Geometry check sheet. Reference: drawing and pictorial views, mm from the part's lowest x, y, z. A direction names the side the tool comes from. Coordinates: 2 decimals unless noted, no trailing zeros. Loops run counter-clockwise (first coordinate to the right, second up) from the corner with the lowest first, then second, coordinate; pieces in that order, holes last. Notation, with made-up numbers: (-29.75, 40.5) -> (-8.75, 40.5) arc R19 cw to (-8.75, 56.5) -> close; hole circle Ø3 at (83.5, 39.25). An arc over 180 degrees is marked (long way). Use CSV: the item, a comma, the result in double quotes.
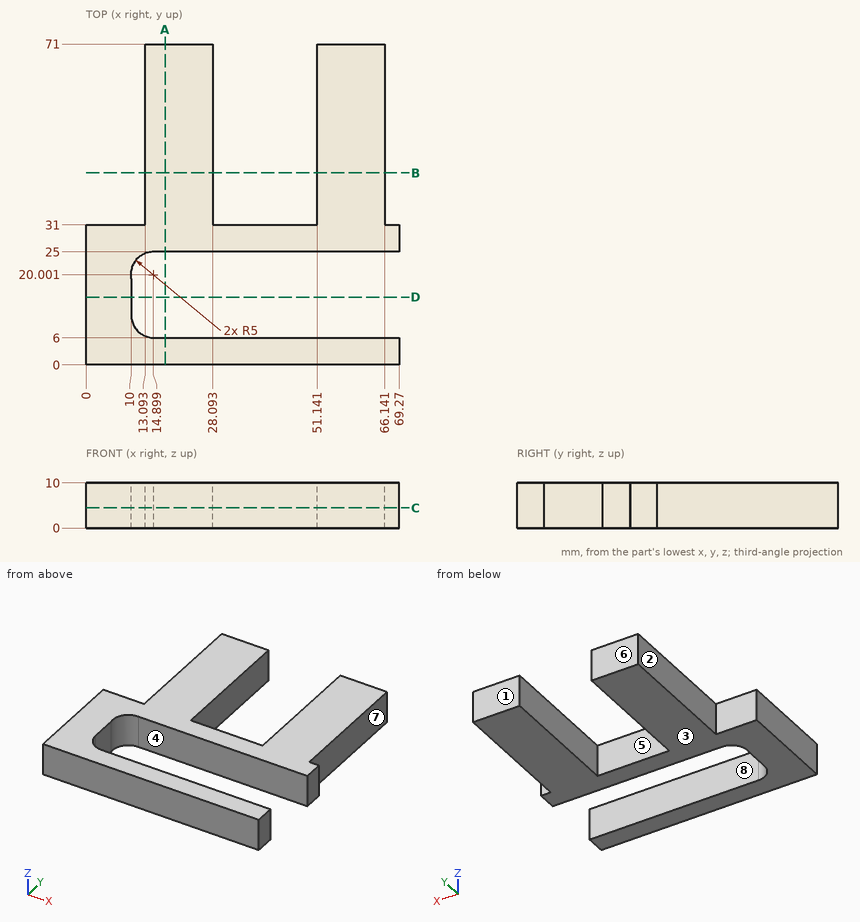
1) Cross-section at C-C on z = 4.5. Record the boundary of the cut face in (x, y), and give its area (3 significant figures).
Answer below:
outline,"(0, 0) -> (69.27, 0) -> (69.27, 6) -> (15, 6) arc R5 cw to (10, 11) -> (10, 19) arc R5 cw to (15, 25) -> (69.27, 25) -> (69.27, 31) -> (66.14, 31) -> (66.14, 71) -> (51.14, 71) -> (51.14, 31) -> (28.09, 31) -> (28.09, 71) -> (13.09, 71) -> (13.09, 31) -> (0, 31) -> close"
area,"2,230 mm²"
2) Cross-section at D-D on y = 15. Record the boundary of the cut face in (x, z), and give its area (3 significant figures).
Answer below:
outline,"(0, 0) -> (10, 0) -> (10, 10) -> (0, 10) -> close"
area,"100 mm²"
3) Access from +Z, -Z, +X, -X, +Y, -Y to the whole of each face (thin tool, end or side, straight path). Record for the marked faces 1, 2, 3, 4 and 5.
Answer below:
face 1,"+Z, -Z, +X, -X, +Y"
face 2,"+Z, -Z, -X, +Y"
face 3,"-Z, +X, -X, +Y, -Y"
face 4,"+Z, -Z, +X"
face 5,"+Z, -Z, +Y"
4) Draft check along Y on the marked faces 6, 7 and 8. Enter one of: released by +Y, released by -Y, zero draft, split by the parting line, or undercut.
Answer below:
face 6,"released by +Y"
face 7,"zero draft"
face 8,"undercut"
5) Go/stop test with flat-tipped pins: pin 1 Ø5 at (x, y) = (28, 22) entering from +Z; pin 2 Ø5 at (y, z) = (53, 6) entering from +X; pin 3 Ø1 at (y, z) = (58.5, 2) entering from -X; pin 4 Ø5 at (x, z) = (9.5, 5.5) entering from +Y. Record where each tip stops, or that it passes through.
Answer below:
pin 1,"passes through"
pin 2,"stops at x = 66.14"
pin 3,"stops at x = 13.09"
pin 4,"stops at y = 31"
6) Cross-section at A-A on x = 17.5. Record the boundary of the cut face in (y, z), and give its area (3 significant figures).
Answer below:
outline,"(0, 0) -> (6, 0) -> (6, 10) -> (0, 10) -> close; (25, 0) -> (71, 0) -> (71, 10) -> (25, 10) -> close"
area,"520 mm²"
7) Thickness scan on line 1 along X through (y, z) = (53.5, 9.5); line 2 along Y through (x, z) = (61.5, 4.5); line 3 along Y through (x, z) = (42, 9.25). Record the ranges inside material, lowest first. Write a range as from..to.
Answer below:
line 1,"x = 13.09..28.09, 51.14..66.14"
line 2,"y = 0..6, 25..71"
line 3,"y = 0..6, 25..31"
8) Cross-section at B-B on y = 42.5. Record the boundary of the cut face in (x, z), and give its area (3 significant figures).
Answer below:
outline,"(13.09, 0) -> (28.09, 0) -> (28.09, 10) -> (13.09, 10) -> close; (51.14, 0) -> (66.14, 0) -> (66.14, 10) -> (51.14, 10) -> close"
area,"300 mm²"
